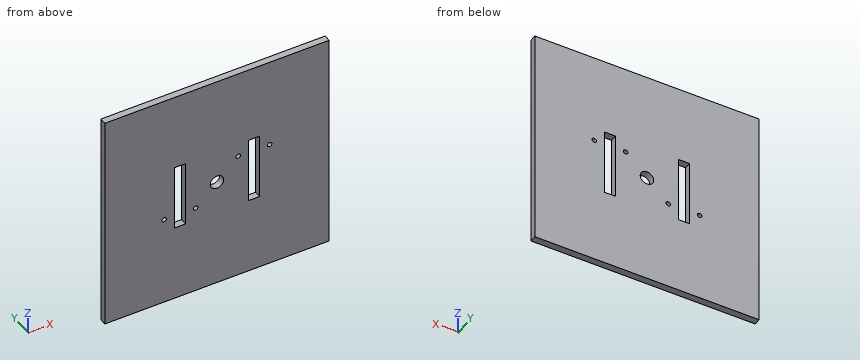
Autodesk Inventor part; units mm, degrees
ref_plane "YZ Plane" through (0, 0, 0) normal (1, 0, 0) x (0, 1, 0)
ref_plane "XZ Plane" through (0, 0, 0) normal (0, 1, 0) x (-1, 0, 0)
ref_plane "XY Plane" through (0, 0, 0) normal (0, 0, 1) x (1, 0, 0)
sketch "Sketch1" plane through (0, 0, 0) normal (0, 1, 0) x (-1, 0, 0)
  line L0 (50, -50) -> (-50, -50)
  line L1 (-50, -50) -> (-50, 50)
  line L2 (-50, 50) -> (50, 50)
  line L3 (50, 50) -> (50, -50)
  line L4 (50, -50) -> (-50, 50) construction
  line L5 (-50, -50) -> (50, 50) construction
  line L6 (-14, -15) -> (-19, -15)
  line L7 (-19, -15) -> (-19, 15)
  line L8 (-19, 15) -> (-14, 15)
  line L9 (-14, 15) -> (-14, -15)
  line L10 (-14, -15) -> (-19, 15) construction
  line L11 (-19, -15) -> (-14, 15) construction
  line L12 (0, -50) -> (0, 50) construction
  line L13 (14, -15) -> (19, -15)
  line L14 (19, -15) -> (19, 15)
  line L15 (19, 15) -> (14, 15)
  line L16 (14, 15) -> (14, -15)
  line L17 (14, -15) -> (19, 15) construction
  line L18 (19, -15) -> (14, 15) construction
  line L19 (-19, 15) -> (-19, 50) construction
  line L20 (-19, -15) -> (-19, -50) construction
  circle A0 centre (0, 0) radius 3
  point P0 (-16.5, 0)
  point P1 (16.5, 0)
  dimension "d0" = 100
  dimension "d1" = 100
  dimension "d4" = 5
  dimension "d5" = 30
  dimension "d6" = 14
  dimension "d21" = 6
extrude "Extrusion2" add sketch "Sketch1" along normal blind 3
sketch "Sketch2" plane through (0, 3, 0) normal (0, 1, 0) x (1, 0, 0)
  circle A0 centre (23.5, -9) radius 1
  circle A1 centre (9.5, -9) radius 1
  line L0 (23.5, -9) -> (16.5, -9) construction
  line L1 (19, -15) -> (14, -15) construction
  line L2 (16.5, -15) -> (16.5, -9) construction
  line L3 (16.5, -9) -> (9.5, -9) construction
  line L4 (-19, 15) -> (-14, 15) construction
  line L5 (-16.5, 15) -> (-16.5, 9) construction
  line L6 (-16.5, 9) -> (-9.5, 9) construction
  line L7 (-16.5, 9) -> (-23.5, 9) construction
  circle A2 centre (-9.5, 9) radius 1
  circle A3 centre (-23.5, 9) radius 1
  point P0 (0, 0)
  dimension "d11" = 2
  dimension "d12" = 2
  dimension "d13" = 6
  dimension "d14" = 7
  dimension "d17" = 2
  dimension "d18" = 2
extrude "Extrusion3" cut sketch "Sketch2" against normal through all
properties part number "thumper-bumper-base"
Verification items for the finished model (mm, model axes). Coordinates: 2 decimals unless noted, no trailing zeros. Loops run counter-clockwise (first coordinate to the right, second up) from the corner with the lowest first, then second, coordinate; pieces in that order, holes last. Notation, with made-up numbers: (-20.5, -13) -> (11.5, -13) arc R21 ccw to (11.5, 8) -> close; hole circle Ø1 at (-33.5, 12.5). An arc over 180 degrees is marked (long way). Answer in a Markdown table with one row per item. Add a question column.
1. Section check D-D, the plane x = -15.5. Enter the section's corners in (y, z).
2. Material ranges on probe 1 along X at (y, z) = (1.2, -11); probe 2 along X at (y, z) = (1.85, -9); probe 3 along X at (y, z) = (1.8, 9), recorded low to high. Write a range as [from, to].
3. Section check A-A, the plane x = 0. Enter the section's corners in (y, z), then the cut area to 3 significant figures.
4. Section check C-C, the plane z = -13.5. Enter the section's corners in (x, y), then the cut area to 3 significant figures.
5. Section check B-B, the plane y = 2.1. Enter the section's corners in (x, z).
Derived:
| question | item | result |
|---|---|---|
| 1 | outline | (0, -50) -> (3, -50) -> (3, -15) -> (0, -15) -> close; (0, 15) -> (3, 15) -> (3, 50) -> (0, 50) -> close |
| 2 | probe 1 | x = [-50, -19], [-14, 14], [19, 50] |
| 2 | probe 2 | x = [-50, -24.5], [-22.5, -19], [-14, -10.5], [-8.5, 14], [19, 50] |
| 2 | probe 3 | x = [-50, -19], [-14, 8.5], [10.5, 14], [19, 22.5], [24.5, 50] |
| 3 | outline | (0, -50) -> (3, -50) -> (3, -3) -> (0, -3) -> close; (0, 3) -> (3, 3) -> (3, 50) -> (0, 50) -> close |
| 3 | area | 282 mm² |
| 4 | outline | (-50, 0) -> (-19, 0) -> (-19, 3) -> (-50, 3) -> close; (-14, 0) -> (14, 0) -> (14, 3) -> (-14, 3) -> close; (19, 0) -> (50, 0) -> (50, 3) -> (19, 3) -> close |
| 4 | area | 270 mm² |
| 5 | outline | (-50, -50) -> (50, -50) -> (50, 50) -> (-50, 50) -> close; hole circle Ø2 at (-23.5, -9); hole (-19, -15) -> (-14, -15) -> (-14, 15) -> (-19, 15) -> close; hole circle Ø2 at (-9.5, -9); hole circle Ø6 at (0, 0); hole circle Ø2 at (9.5, 9); hole (14, -15) -> (19, -15) -> (19, 15) -> (14, 15) -> close; hole circle Ø2 at (23.5, 9) |
